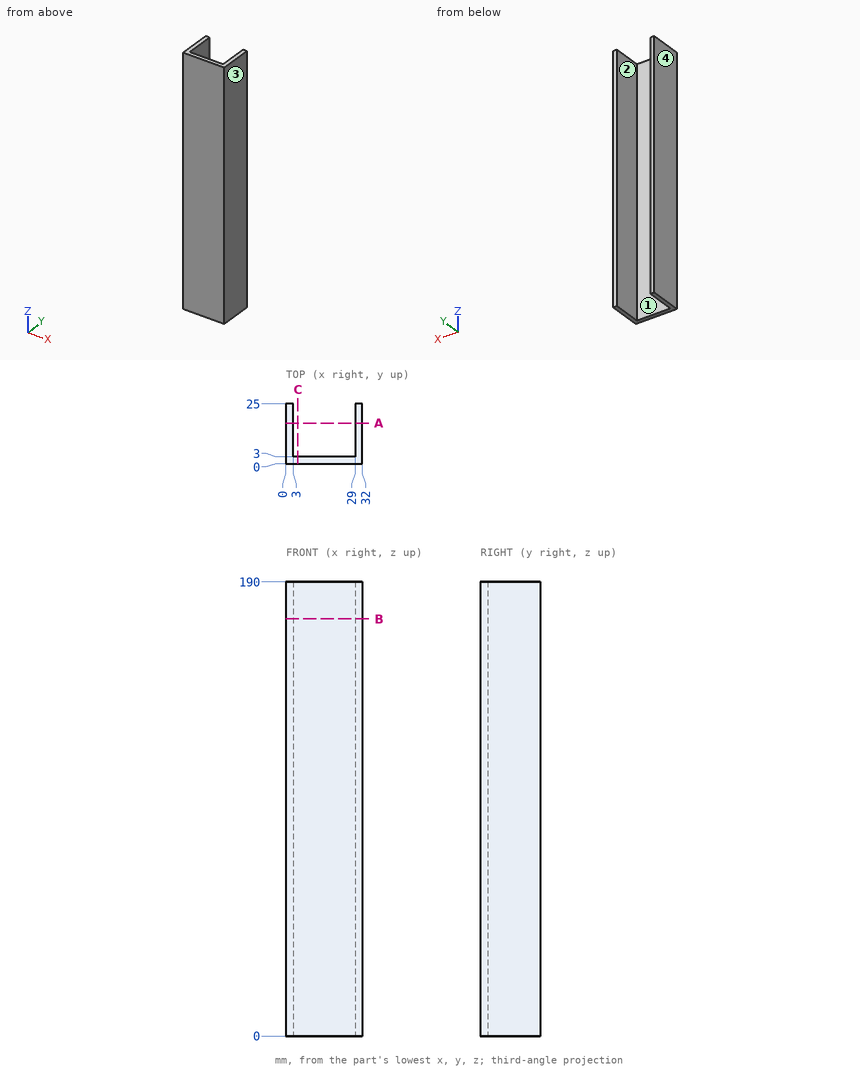
The figure shows three views and two pictorial views of one solid part (mm, origin at its lowest corner). Answer the questions. Coordinates: 2 decimals unless noted, no trailing zeros. Order: outer loops, then holes, each group sorted by start corner. A loop starts at its lowest first (then second) coordinate and runs counter-clockwise, first axis right, second up. Notation, with made-up numbers: M 42.5,25 L 96.5,25 A23 ccw 96.5,47 Z; hole C 0.5,-1 d3. An arc over 180 degrees is marked long. Use CSV: the item, a comma, the result in double quotes.
1) Determine the mould class of the marked faces 1, 2, 3 and 4 for opening direction X: released by +X, released by -X, zero draft, split by the parting line, or undercut.
Worked out:
face 1,"undercut"
face 2,"undercut"
face 3,"released by +X"
face 4,"released by -X"
2) Consider line 1 (X direction, y = 21, z = 53); line 2 (Y direction, x = 25, z = 145.5). Determine where each line is inside the solid, lowest interval first. Write a range as [from, to].
Worked out:
line 1,"x = [0, 3], [29, 32]"
line 2,"y = [0, 3]"
3) Flat-ended cylindrical pins translate along their axes: pin 1 Ø6 at (x, z) = (3.5, 31.5) entering from -Y; pin 2 Ø8 at (x, z) = (12, 74.5) entering from +Y. Find the tip coordinate at first contact, or state that the pin passes through.
Worked out:
pin 1,"stops at y = 0"
pin 2,"stops at y = 3"
4) Section C-C on x = 5 is taken. Write down the section's boundary in (y, z).
Worked out:
outline,"M 0,0 L 3,0 L 3,190 L 0,190 Z"
5) Section B-B on z = 174.5 is taken. Write down the section's boundary in (x, y), plus the area to 3 significant figures.
Worked out:
outline,"M 0,0 L 32,0 L 32,25 L 29,25 L 29,3 L 3,3 L 3,25 L 0,25 Z"
area,"228 mm^2"
6) Section A-A on y = 17 is taken. Write down the section's boundary in (x, z), plus the area to 3 significant figures.
Worked out:
outline,"M 0,0 L 3,0 L 3,190 L 0,190 Z; M 29,0 L 32,0 L 32,190 L 29,190 Z"
area,"1,140 mm^2"
